Geometry: final body of the model. Coordinates: model frame, mm. Round coordinates to 2 decimals unless told otherwise and drop trailing zeros. Loops run counter-clockwise (first coordinate to the right, second up) from the corner with the lowest first, then second, coordinate; pieces in that order, holes last. Notation, with made-up numbers: (32.25, 69) -> (50.25, 69) arc R7 ccw to (50.25, 73) -> close; hole circle Ø8 at (63, -32). An arc over 180 degrees is marked (long way). Answer in a Markdown table with one row per item.
```python
from build123d import *

# Parameters (mm, degrees)
BOSS_EXTRUDE1_DEPTH = 12.7
SKETCH2_R           = 6.35
CUT_EXTRUDE1_DEPTH  = 522.473815258
SKETCH3_W           = 76.2
SKETCH3_H           = 38.1
BOSS_EXTRUDE4_DEPTH = 25.4
SKETCH6_W           = 66.675
SKETCH6_H           = 25.4
CUT_EXTRUDE3_DEPTH  = 522.667089723
SKETCH4_R           = 6.35
CUT_EXTRUDE2_DEPTH  = 523.246483952
FILLET3_R           = 3.175


with BuildPart() as part:
    # Sketch1 → Boss-Extrude1 (new, symmetric)
    with BuildSketch(Plane.XY):
        with BuildLine():
            Line((-508, 12.7), (508, 12.7))
            ThreePointArc((508, 12.7), (520.7, 0), (508, -12.7))
            Line((508, -12.7), (-508, -12.7))
            ThreePointArc((-508, -12.7), (-520.7, 0), (-508, 12.7))
        make_face()
    extrude(amount=BOSS_EXTRUDE1_DEPTH, both=True)

    # Sketch2 → Cut-Extrude1 (cut, through all)
    with BuildSketch(Plane.XY.offset(12.7)):
        with Locations((-508, 0)):
            Circle(SKETCH2_R)
        with Locations((508, 0)):
            Circle(SKETCH2_R)
    extrude(amount=-CUT_EXTRUDE1_DEPTH, mode=Mode.SUBTRACT)

    # Sketch3 → Boss-Extrude4 (add, through all)
    with BuildSketch(Plane(origin=(0, 12.7, 0), x_dir=(1, 0, 0), z_dir=(0, 1, 0))):
        with Locations((482.6, 0)):
            Rectangle(SKETCH3_W, SKETCH3_H)
    extrude(amount=-BOSS_EXTRUDE4_DEPTH)

    # Sketch6 → Cut-Extrude3 (cut, through all)
    with BuildSketch(Plane(origin=(0, 12.7, 0), x_dir=(1, 0, 0), z_dir=(0, 1, 0))):
        with Locations((487.3625, 0)):
            Rectangle(SKETCH6_W, SKETCH6_H)
    extrude(amount=-CUT_EXTRUDE3_DEPTH, mode=Mode.SUBTRACT)

    # Sketch4 → Cut-Extrude2 (cut, through all)
    with BuildSketch(Plane.XY.offset(19.05)):
        with BuildLine():
            Line((520.7, 0), (520.7, 12.7))
            Line((520.7, 12.7), (508, 12.7))
            ThreePointArc((508, 12.7), (516.980256121, 8.980256121), (520.7, 0))
        make_face()
        with BuildLine():
            Line((520.7, -12.7), (520.7, 0))
            ThreePointArc((520.7, 0), (516.980256121, -8.980256121), (508, -12.7))
            Line((508, -12.7), (520.7, -12.7))
        make_face()
        with Locations((508, 0)):
            Circle(SKETCH4_R)
    extrude(amount=-CUT_EXTRUDE2_DEPTH, mode=Mode.SUBTRACT)

    # Fillet3
    fillet3_edges = [part.edges().sort_by_distance(p)[0] for p in [
        (454.025, 0, 12.7),
        (444.5, 0, -19.05),
        (444.5, 0, -12.7),
        (444.5, 0, 12.7),
        (454.025, 0, -12.7),
        (444.5, 0, 19.05),
    ]]
    fillet(fillet3_edges, radius=FILLET3_R - 0.0001)  # a hair under: the kernel refuses the full size


solid = part.part
```
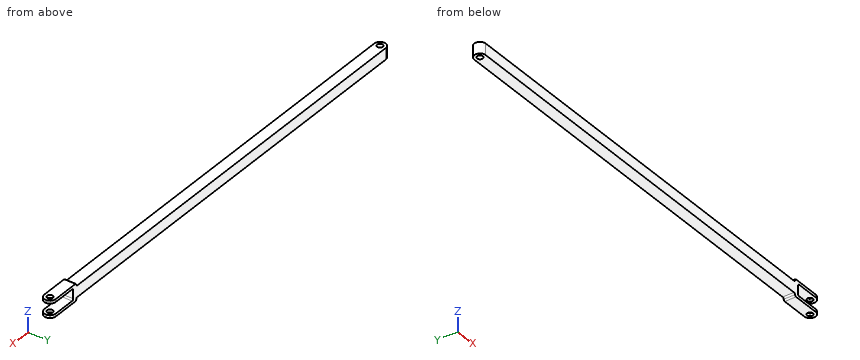
Item 1: Section query A-A, the plane z = 1.5. Output: boundary loops of the cut face in (x, y) (3 decimals), and give its area (3 significant figures).
Ans:
| item | result |
|---|---|
| outline | (-508, -12.7) -> (454.025, -12.7) -> (454.025, 12.7) -> (-508, 12.7) arc R12.7 ccw to start; hole circle Ø12.7 at (-508, 0) |
| area | 24,600 mm2 |
Item 2: Section query B-B, the plane x = 178. Output: boundary loops of the cut face in (y, z).
Ans:
| item | result |
|---|---|
| outline | (-12.7, -12.7) -> (12.7, -12.7) -> (12.7, 12.7) -> (-12.7, 12.7) -> close |
Item 3: Ray query, L1, parallel to X at y = 0.5, z = 16; L2, parallel to Y at x = -508, z = -7; L3, parallel to X at y = -0.25, z = 1.5 (3 decimals). Return the intervals inside material, ascending.
Ans:
| item | result |
|---|---|
| L1 | 444.5 to 501.67, 514.33 to 520.69 |
| L2 | -12.7 to -6.35, 6.35 to 12.7 |
| L3 | -520.698 to -514.345, -501.655 to 454.025 |
Item 4: First-contact query: P1, Ø1.5, axis at x = 169, y = 7, coming from the -Z side; P2, Ø3, axis at y = -8.5, z = -6.5, coming from the -X side; P3, Ø11.5, axis at x = 508, y = 0, coming from the -Z side; P4, Ø1.5, axis at x = 9.5, y = -0.5, coming from the +Z side. Flat tips, straight axial feed; report the tip coordinate or a pass-through.
Ans:
| item | result |
|---|---|
| P1 | z = -12.7 |
| P2 | x = -518.6 |
| P3 | through |
| P4 | z = 12.7 |
